Input: part model. Units: mm. Frame: model coordinates. Round coordinates to 2 decimals unless told otherwise and drop trailing zeros. Loops run counter-clockwise (first coordinate to the right, second up) from the corner with the lowest first, then second, coordinate; pieces in that order, holes last. Notation, with made-up numbers: (11, 44) -> (48, 44) arc R28 ccw to (48, 77) -> close; hole circle Ø10 at (-33.5, -39). An arc over 180 degrees is marked (long way). One line per question, with ' | ' between items. Start each with the question number.
Q1. Material intervals for L1, parallel to X at y = 17, z = 0.65; L2, parallel to X at y = 25.5, z = 2.65; L3, parallel to X at y = 73, z = 0.5, sorted ascending.
Q2. Contact query for a flat-ended pin moving along its axis: P1, Ø2, axis at x = 25, y = 33.5, coming from the -Z side. Output: stop coordinate, or through.
Q3. Cut plane A-A on x = 52.5. Return loops of the section in (y, z), and give its area (3 significant figures).
Q4. Cut plane B-B on z = 0.95. State how many separate pieces and enclosed holes the cut face has, and give its area (3 significant figures).
from build123d import *

# Parameters (mm, degrees)
SKETCH_W        = 76.2
SKETCH_H        = 169.6
PAD_DEPTH       = 2.8
SKETCH001_W     = 13.9993
SKETCH001_H     = 13.9993
SKETCH001_H_2   = 13.99946
SKETCH001_W_2   = 13.99955
SKETCH001_H_3   = 13.9994
POCKET_DEPTH    = 5
SKETCH002_R     = 1.6
POCKET001_DEPTH = 2.801
SKETCH011_R     = 0.95
POCKET002_DEPTH = 2.801


with BuildPart() as part:
    # Sketch → Pad (new body)
    with BuildSketch(Plane.XY):
        with Locations((38.1, 84.8)):
            Rectangle(SKETCH_W, SKETCH_H)
    extrude(amount=PAD_DEPTH)

    # Sketch001 (on Face6 of Pad) → Pocket (cut)
    with BuildSketch(Plane.XY.offset(2.8)):
        with Locations((66.674265, 85.725757)):
            Rectangle(SKETCH001_W, SKETCH001_H)
        with Locations((47.624265, 85.725757)):
            Rectangle(SKETCH001_W, SKETCH001_H)
        Polygon((5.498385, 17.495607), (5.499755, 16.295307), (3.774465, 16.295307), (3.774465, 10.025207), (2.949005, 10.025207), (2.949005, 7.225037), (3.774465, 7.225037), (3.774465, 3.994937), (10.524115, 3.994937), (10.524115, 7.225037), (12.049615, 7.225037), (12.049615, 2.525947), (26.049015, 2.525947), (26.049015, 7.225037), (27.574515, 7.225037), (27.574515, 3.994937), (34.324215, 3.994937), (34.324215, 7.225037), (35.149615, 7.225037), (35.149615, 10.025207), (34.324215, 10.025207), (34.324215, 16.295307), (32.598915, 16.295307), (32.598915, 17.495607), (29.299815, 17.495607), (29.299815, 16.295307), (27.574515, 16.295307), (27.574515, 11.824907), (26.049015, 11.824907), (26.049015, 16.525407), (12.049615, 16.525407), (12.049615, 11.824907), (10.524115, 11.824907), (10.524115, 16.295307), (8.798765, 16.295307), (8.798765, 17.495607), align=None)
        with Locations((47.624265, 9.525677)):
            Rectangle(SKETCH001_W, SKETCH001_H_2)
        Polygon((64.375015, 35.151007), (64.375015, 34.325607), (61.145015, 34.325607), (61.145015, 27.575907), (64.375015, 27.575907), (64.375015, 26.050407), (59.674615, 26.050407), (59.674615, 12.050907), (64.375015, 12.050907), (64.375015, 10.525407), (61.145015, 10.525407), (61.145015, 3.775827), (64.375015, 3.775827), (64.375015, 2.950377), (67.174015, 2.950377), (67.174015, 3.775827), (73.443915, 3.775827), (73.443915, 5.501117), (74.644015, 5.501117), (74.644015, 8.800157), (73.443915, 8.800157), (73.443915, 10.525407), (68.974915, 10.525407), (68.974915, 12.050907), (73.673915, 12.050907), (73.673915, 26.050407), (68.974915, 26.050407), (68.974915, 27.575907), (73.443915, 27.575907), (73.443915, 29.301207), (74.644015, 29.301207), (74.644015, 32.600207), (73.443915, 32.600207), (73.443915, 34.325607), (67.174015, 34.325607), (67.174015, 35.151007), align=None)
        with Locations((9.52434, 28.575607)):
            Rectangle(SKETCH001_W_2, SKETCH001_H_3)
        with Locations((28.574265, 28.575607)):
            Rectangle(SKETCH001_W, SKETCH001_H_3)
        with Locations((47.624265, 28.575607)):
            Rectangle(SKETCH001_W, SKETCH001_H_3)
        with Locations((9.52434, 47.625757)):
            Rectangle(SKETCH001_W_2, SKETCH001_H)
        with Locations((28.574265, 47.625757)):
            Rectangle(SKETCH001_W, SKETCH001_H)
        with Locations((47.624265, 47.625757)):
            Rectangle(SKETCH001_W, SKETCH001_H)
        Polygon((64.375015, 73.251007), (64.375015, 72.425507), (61.145015, 72.425507), (61.145015, 65.675807), (64.375015, 65.675807), (64.375015, 64.150407), (59.674615, 64.150407), (59.674615, 50.151107), (64.375015, 50.151107), (64.375015, 48.625307), (61.145015, 48.625307), (61.145015, 41.876007), (64.375015, 41.876007), (64.375015, 41.050507), (67.174015, 41.050507), (67.174015, 41.876007), (73.443915, 41.876007), (73.443915, 43.601007), (74.644015, 43.601007), (74.644015, 46.900207), (73.443915, 46.900207), (73.443915, 48.625307), (68.974915, 48.625307), (68.974915, 50.151107), (73.673915, 50.151107), (73.673915, 64.150407), (68.974915, 64.150407), (68.974915, 65.675807), (73.443915, 65.675807), (73.443915, 67.401207), (74.644015, 67.401207), (74.644015, 70.701807), (73.443915, 70.700407), (73.443915, 72.425507), (67.174015, 72.425507), (67.174015, 73.251007), align=None)
        with Locations((9.52434, 66.675757)):
            Rectangle(SKETCH001_W_2, SKETCH001_H)
        with Locations((28.574265, 66.675757)):
            Rectangle(SKETCH001_W, SKETCH001_H)
        with Locations((47.624265, 66.675757)):
            Rectangle(SKETCH001_W, SKETCH001_H)
        with Locations((9.52434, 85.725757)):
            Rectangle(SKETCH001_W_2, SKETCH001_H)
        with Locations((28.574265, 85.725757)):
            Rectangle(SKETCH001_W, SKETCH001_H)
    extrude(amount=-POCKET_DEPTH, mode=Mode.SUBTRACT)

    # Sketch002 (on Face5 of Pocket) → Pocket001 (cut, through all)
    with BuildSketch(Plane.XY.offset(2.8)):
        with Locations((19.049365, 57.150757)):
            Circle(SKETCH002_R)
        with Locations((57.149265, 76.200757)):
            Circle(SKETCH002_R)
        with Locations((57.149265, 38.100707)):
            Circle(SKETCH002_R)
        with Locations((4, 97.25)):
            Circle(SKETCH002_R)
        with Locations((72.2, 97.25)):
            Circle(SKETCH002_R)
    extrude(amount=-POCKET001_DEPTH, mode=Mode.SUBTRACT)

    # Sketch011 (on Face5 of Pocket001) → Pocket002 (cut, through all)
    with BuildSketch(Plane.XY.offset(2.8)):
        with Locations((4.6, 125)):
            Circle(SKETCH011_R)
        with Locations((71.6, 125)):
            Circle(SKETCH011_R)
        with Locations((4.6, 165)):
            Circle(SKETCH011_R)
        with Locations((71.6, 165)):
            Circle(SKETCH011_R)
    extrude(amount=-POCKET002_DEPTH, mode=Mode.SUBTRACT)


solid = part.part
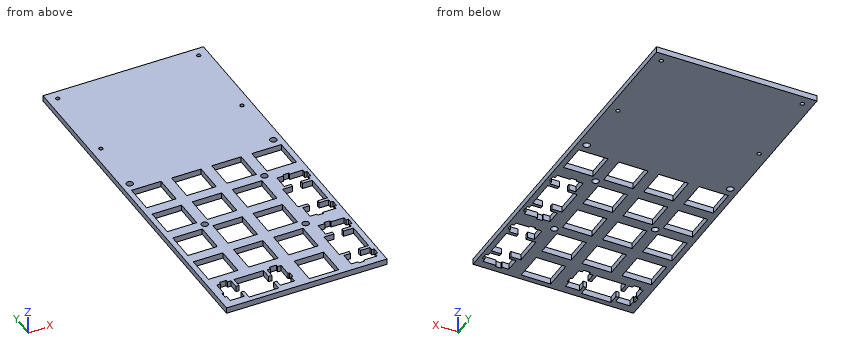
Results:
1) L1: 0 to 5.5, 8.8 to 29.3, 32.6 to 59.67, 73.67 to 76.2 | L2: 0 to 2.52, 16.52 to 21.57, 35.57 to 40.62, 54.62 to 59.67, 73.67 to 76.2 | L3: 0 to 2.52, 16.52 to 21.57, 35.57 to 40.62, 54.62 to 64.38, 67.17 to 76.2
2) P1: through
3) outline: (0, 0) -> (2.53, 0) -> (2.53, 2.8) -> (0, 2.8) -> close; (16.53, 0) -> (21.58, 0) -> (21.58, 2.8) -> (16.53, 2.8) -> close; (35.58, 0) -> (40.63, 0) -> (40.63, 2.8) -> (35.58, 2.8) -> close; (54.63, 0) -> (59.68, 0) -> (59.68, 2.8) -> (54.63, 2.8) -> close; (73.68, 0) -> (78.73, 0) -> (78.73, 2.8) -> (73.68, 2.8) -> close; (92.73, 0) -> (169.6, 0) -> (169.6, 2.8) -> (92.73, 2.8) -> close | area: 279 mm^2
4) separate pieces: 1 | enclosed holes: 26 | area: 8,960 mm^2
